CAD build for the part. Positions are in the model's coordinates, mm. A direction names the side the tool comes from. Coordinates: 2 decimals unless noted, no trailing zeros. Loops run counter-clockwise (first coordinate to the right, second up) from the corner with the lowest first, then second, coordinate; pieces in that order, holes last. Notation, with made-up numbers: (9.25, -27.75) -> (14.25, -27.75) arc R26 cw to (14.25, -1.75) -> close; hole circle Ø1 at (80.5, 80). An arc over 180 degrees is marked (long way). Return JSON: item names as keys, results as strings. Group by question number.
(1) Mould opens along Z. For faces 1 (the face through (-3, 7.45, 3)), 2 (the face through (-2.72, 2.46, -1.54)), 3 (the face through (-3.89, 4.18, -5.08)) say: pulls with the +Z half, pulls with the -Z half, needs draft (parallel to the pull), parting line crosses it, or undercut.
(2) Flat gauge pins, fed straight in: pin 1 Ø7 at (x, z) = (0, -0.5) entering from -Y; pin 2 Ø1 at (x, y) = (-0.5, 44) entering from +Z (3 decimals); pin 3 Ø6 at (y, z) = (56.5, 0) entering from -X (3 decimals); pin 4 Ø2 at (y, z) = (60.5, 3.5) entering from +X. Where does each tip first touch, or does it go through?
(3) Saw through at B-B on y = 9. Write the cut outline in (x, z) (3 decimals).
(4) Tool access for faces 4 (the face through (0, 107.45, 0)), 5 (the face through (-2.694, 2.465, 1.584)), 6 (the face through (-3.685, 56.75, -0.818)): list every direction of +Z, -Z, +X, -X, +Y, -Y with a clear straight run to the whole face (end or side of a thin tool).
(5) Probe L1, parallel to X at y = 41, z = -0.25; L2, parallel to Y at x = -2.5, z = -3; L3, parallel to Y at x = -1, z = 1. List the from-to ranges inside material, lowest first.
(6) Saw through at A-A on x = 0. Write the cut outline in (y, z) (3 decimals).
```python
from build123d import *

# Parameters (mm, degrees)
SKETCH1_R           = 6.4
BOSS_EXTRUDE1_DEPTH = 7.45
SKETCH2_R           = 3.775
BOSS_EXTRUDE2_DEPTH = 100
CUT_EXTRUDE1_DEPTH  = 5


with BuildPart() as part:
    # Sketch1 → Boss-Extrude1 (new body)
    with BuildSketch(Plane(origin=(0, 0, 0), x_dir=(1, 0, 0), z_dir=(0, 1, 0))):
        with Locations(Location((0, 0, 0), (0, 0, 270))):
            Circle(SKETCH1_R)
    extrude(amount=BOSS_EXTRUDE1_DEPTH)

    # Sketch2 → Boss-Extrude2 (add)
    with BuildSketch(Plane(origin=(0, 7.45, 0), x_dir=(1, 0, 0), z_dir=(0, 1, 0))):
        with Locations(Location((0, 0, 0), (0, 0, 270))):
            Circle(SKETCH2_R)
    extrude(amount=BOSS_EXTRUDE2_DEPTH)

    # Sketch3 → Cut-Extrude1 (cut)
    with BuildSketch(Plane.XZ):
        Polygon((-3.608439182, 0), (-1.804219591, -3.125), (1.804219591, -3.125), (3.608439182, 0), (1.804219591, 3.125), (-1.804219591, 3.125), align=None)
    extrude(amount=-CUT_EXTRUDE1_DEPTH, mode=Mode.SUBTRACT)

    # Sketch4 → Cut-Revolve1 (revolve, cut)
    with BuildSketch(Plane(origin=(0, 0, 0), x_dir=(0, 0, -1), z_dir=(1, 0, 0))):
        Polygon((5.4, 0), (6.4, 1), (6.4, 0), align=None)
    revolve(axis=Axis((0, 0, 0), (0, 1, 0)), mode=Mode.SUBTRACT)


solid = part.part
```
Geometry results:
{
 "1": {"face 1": "needs draft", "face 2": "undercut", "face 3": "parting line crosses it"},
 "2": {"pin 1": "y = 0", "pin 2": "z = 3.775", "pin 3": "x = -3.775", "pin 4": "x = 2.83"},
 "3": {"outline": "circle Ø7.55 at (0, 0)"},
 "4": {"face 4": "+Z, -Z, +X, -X, +Y", "face 5": "-Y", "face 6": "+Y"},
 "5": {"L1": "-3.77 to 3.77", "L2": "0 to 7.45", "L3": "5 to 107.45"},
 "6": {"outline": "(0, -5.4) -> (1, -6.4) -> (7.45, -6.4) -> (7.45, -3.775) -> (107.45, -3.775) -> (107.45, 3.775) -> (7.45, 3.775) -> (7.45, 6.4) -> (1, 6.4) -> (0, 5.4) -> (0, 3.125) -> (5, 3.125) -> (5, -3.125) -> (0, -3.125) -> close"}
}
